Design review of the part built by this model. Coordinates are the model's own, in mm. Coordinates: 2 decimals unless noted, no trailing zeros. Loops run counter-clockwise (first coordinate to the right, second up) from the corner with the lowest first, then second, coordinate; pieces in that order, holes last.
Autodesk Inventor part; units mm, degrees
ref_plane "YZ Plane" through (0, 0, 0) normal (1, 0, 0) x (0, 1, 0)
ref_plane "XZ Plane" through (0, 0, 0) normal (0, 1, 0) x (-1, 0, 0)
ref_plane "XY Plane" through (0, 0, 0) normal (0, 0, 1) x (1, 0, 0)
ref_plane "작업 평면1" through (0, 0, 0) normal (0, 0, 1) x (1, 0, 0)
ref_plane "작업 평면2" through (0, 0, 0) normal (0, 0, 1) x (1, 0, 0)
sketch "스케치2" plane through (0, 0, 0) normal (0, 0, 1) x (1, 0, 0)
  circle A0 centre (-53.6, -73.63) radius 1.35
  circle A1 centre (-62.8, -73.63) radius 1.35
  line L0 (-72, -70.63) -> (-44.4, -70.63)
  line L1 (-72, -70.63) -> (-72, -76.63)
  line L2 (-72, -76.63) -> (-44.4, -76.63)
  line L3 (-44.4, -70.63) -> (-44.4, -76.63)
  circle A2 centre (18.4, -73.63) radius 1.35
  circle A3 centre (9.2, -73.63) radius 1.35
  line L4 (0, -70.63) -> (27.6, -70.63)
  line L5 (0, -70.63) -> (0, -76.63)
  line L6 (0, -76.63) -> (27.6, -76.63)
  line L7 (27.6, -70.63) -> (27.6, -76.63)
  circle A4 centre (18.4, -3) radius 1.35
  circle A5 centre (8.5755, -3) radius 1.35
  line L8 (0, 0) -> (27.6, 0)
  line L9 (0, 0) -> (0, -6)
  line L10 (0, -6) -> (27.6, -6)
  line L11 (27.6, 0) -> (27.6, -6)
  circle A6 centre (-62.8, -3) radius 1.35
  circle A7 centre (-52.9755, -3) radius 1.35
  line L12 (-44.4, 0) -> (-72, 0)
  line L13 (-72, 0) -> (-72, -6)
  line L14 (-44.4, -6) -> (-72, -6)
  line L15 (-44.4, 0) -> (-44.4, -6)
  line L16 (27.6, 0) -> (27.6, -76.63)
  line L17 (27.6, -76.63) -> (-72, -76.63)
  line L18 (-72, -76.63) -> (-72, 0)
  line L19 (-72, 0) -> (27.6, 0)
  point P0 (27.6, -70.63)
  point P1 (27.6, -6)
extrude "돌출1" add sketch "스케치2" along normal blind 6
sketch "스케치3" plane through (0, 0, 6) normal (0, 0, 1) x (1, 0, 0)
  line L0 (-72, -76.63) -> (27.6, -76.63)
  line L1 (27.6, 0) -> (-72, 0)
  line L2 (-72, -76.63) -> (-72, 0)
  line L3 (-72, 0) -> (-72, -42.4915)
  line L4 (-22.2, -76.63) -> (-22.2, 0)
  line L5 (-72, -38.315) -> (27.6, -38.315)
  circle A0 centre (-22.2, -38.315) radius 5
  point P0 (0, 0)
  dimension "d3" = 10
extrude "돌출2" cut sketch "스케치3" against normal blind 6 contours A0 L5 L4 | L4 L5 A0 | L5 A0 L4 | L4 A0 L5
sketch "스케치4" plane through (0, 0, 6) normal (0, 0, 1) x (1, 0, 0)
  circle A0 centre (-22.2, -38.315) radius 13.9
  circle A1 centre (-25.6914, -27.8838) radius 1.25
  circle A2 centre (-32.0448, -33.4078) radius 1.55
  circle A3 centre (-17.2928, -28.4702) radius 1.25
  circle A4 centre (-11.7688, -34.8236) radius 1.25
  circle A5 centre (-12.3552, -43.2222) radius 1.25
  circle A6 centre (-18.7086, -48.7462) radius 1.55
  circle A7 centre (-27.1072, -48.1598) radius 1.55
  circle A8 centre (-32.6312, -41.8064) radius 1.55
  circle A9 centre (-25.6914, -27.8838) radius 1.55
  circle A10 centre (-17.2928, -28.4702) radius 1.55
  circle A11 centre (-11.7688, -34.8236) radius 1.55
  circle A12 centre (-12.3552, -43.2222) radius 1.55
  circle A13 centre (-32.6312, -41.8064) radius 1.25
  circle A14 centre (-27.1072, -48.1598) radius 1.25
  circle A15 centre (-18.7086, -48.7462) radius 1.25
  circle A16 centre (-32.0448, -33.4078) radius 1.25
  point P0 (0, 0)
extrude "돌출3" cut sketch "스케치4" against normal blind 6 contours A1 | A2 | A3 | A4 | A5 | A6 | A7 | A8 | A9 | A10 | A11 | A12 | A13 | A14 | A15 | A16
fillet "모깎기1" radius 2 4 edges at (-72, 0, 3) (27.6, 0, 3) (27.6, -76.63, 3) (-72, -76.63, 3)
properties part number "_pelvis" material "PMMA 플라스틱"
Q1. Take a section at B-B, the plane x = -22.2. Write out the cut boundary in (y, z) (3 decimals).
Q2. Take a section at A-A, the plane x = 18.4. Write out the cut boundary in (y, z).
Q3. For line 1 (Y direction, x = -62.8, z = 3.55); line 2 (X direction, y = -73.63, z = 4.65); line 3 (Y direction, x = -22.2, z = 2.85) (3 decimals), list the stretches that pass through material, from the lowest coordinate up.
Q4. The part is to be moulded in two halves that separate along X. For faces 1 (the cylindrical face through (27, -76.06, 3.04)), 2 (the flat face through (-23, -29, 0)), 3 (the cylindrical face through (-19.04, -50.26, 3.04)), say which applies: pulls with the +X half, pulls with the -X half, needs draft (parallel to the pull), parting line crosses it, or undercut.
Q5. Take a section at C-C, the plane z = 2.2. Give the number of separate pieces and of enclosed holes in the cut face, then the cut area to 3 significant figures.
Q6. Clearance check with flat-ended pins moving along their axes: pin 1 Ø4 at (x, y) = (-11.77, -34.82) entering from +Z; pin 2 Ø1.6 at (x, y) = (18.4, -3) entering from +Z (3 decimals). State where each tip first meets the part, or that it passes through.
Entries:
1. outline: (-76.63, 0) - (-43.315, 0) - (-43.315, 6) - (-76.63, 6) - close; (-33.315, 0) - (0, 0) - (0, 6) - (-33.315, 6) - close
2. outline: (-76.63, 0) - (-74.98, 0) - (-74.98, 6) - (-76.63, 6) - close; (-72.28, 0) - (-4.35, 0) - (-4.35, 6) - (-72.28, 6) - close; (-1.65, 0) - (0, 0) - (0, 6) - (-1.65, 6) - close
3. line 1: y = -76.63 to -74.98, -72.28 to -4.35, -1.65 to 0
3. line 2: x = -72 to -64.15, -61.45 to -54.95, -52.25 to 7.85, 10.55 to 17.05, 19.75 to 27.6
3. line 3: y = -76.63 to -43.315, -33.315 to 0
4. face 1: pulls with the +X half
4. face 2: needs draft
4. face 3: undercut
5. separate pieces: 1
5. enclosed holes: 17
5. area: 7,440 mm2
6. pin 1: stops at z = 6
6. pin 2: passes through
